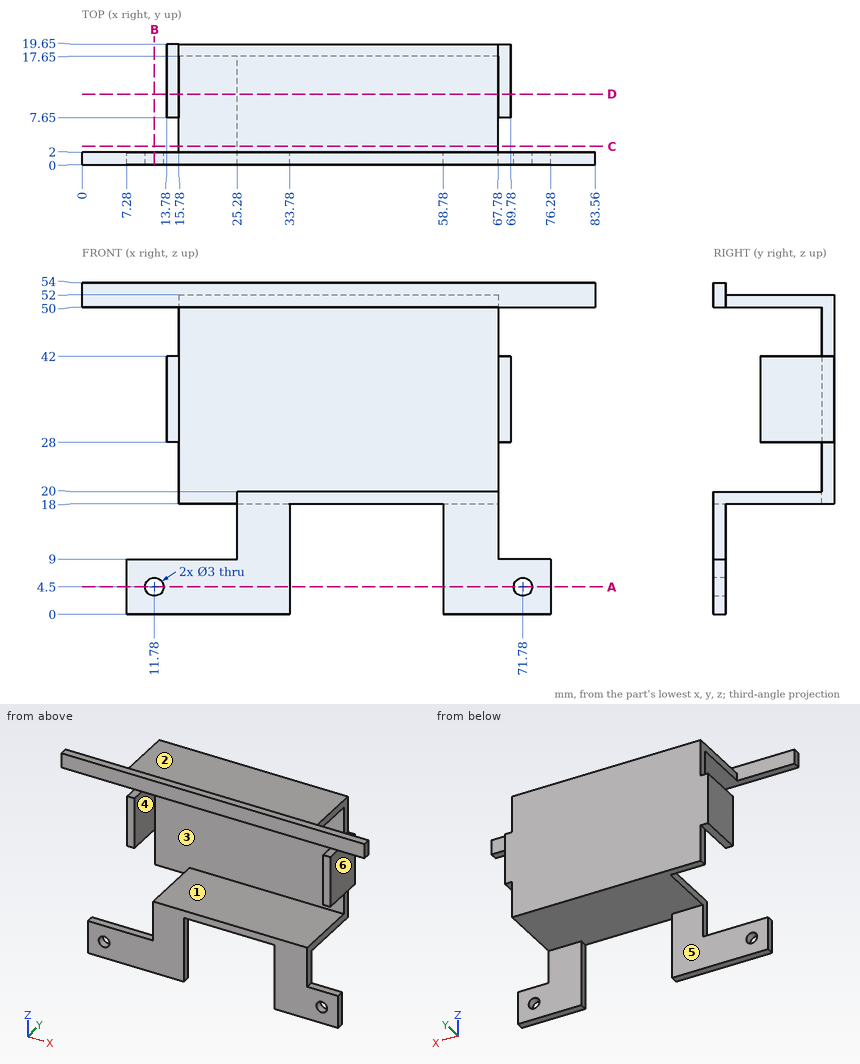
Design review of the part shown in the three views and the two pictorial views. Dimensions are in mm from the part's minimum x, y and z. A direction names the side the tool comes from. Coordinates: 2 decimals unless noted, no trailing zeros. Write each loop counter-clockwise with the first axis right and the second up, starting at its lowest first coordinate (ties: lowest second). Pieces come first, ordered by that corner, then holes.
(1) The part is to be moulded in two halves that separate along Z. For the marked faces 1, 2, 3 and 4, say which applies: +Z half, -Z half, draft (parallel to the pull), parting line (faces both ways), or undercut.
(2) Add section B-B on x = 11.78. Give the boundary of the cut face in (y, z), then the cut area to 3 significant figures.
(3) Add section D-D on y = 11.5. Give the boundary of the cut face in (x, z), then the cut area to 3 significant figures.
(4) Add section A-A on z = 4.5. Give the boundary of the cut face in (x, y).
(5) Add section C-C on y = 3. Give the boundary of the cut face in (x, z), then the cut area to 3 significant figures.
(6) Wall thickness on probe 1 along Z at (x, y) = (71.78, 1.1); probe 2 along X at (y, z) = (0.5, 4.5); probe 3 along Z at (x, y) = (14.5, 1): over which ranges is each line inside the solid? List them lowest first.
(7) Tool access review of the marked faces 5 and 6: name each direction out of +Z, -Z, +X, -X, +Y, -Y from which nothing blocks a thin tool from reaching the whole face with its end or side.
(8) For pin 1 Ø3 at (y, z) = (7, 35.5) entering from -X; pin 2 Ø6 at (x, z) = (18.5, 18) entering from -Y; pin 3 Ø2 at (x, z) = (14.5, 46.5) entering from +Y; pin 4 Ø2 at (x, z) = (15, 36) entering from -Y, all flat-tipped, find the tip position at first contact; note any pin that passes through.
Answer sheet:
1. face 1: undercut
1. face 2: +Z half
1. face 3: undercut
1. face 4: draft
2. outline: (0, 0) - (2, 0) - (2, 3) - (0, 3) - close; (0, 6) - (2, 6) - (2, 9) - (0, 9) - close; (0, 50) - (2, 50) - (2, 54) - (0, 54) - close
2. area: 20.0 mm2
3. outline: (13.78, 28) - (15.78, 28) - (15.78, 42) - (13.78, 42) - close; (15.78, 50) - (67.78, 50) - (67.78, 52) - (15.78, 52) - close; (25.28, 18) - (67.78, 18) - (67.78, 20) - (25.28, 20) - close; (67.78, 28) - (69.78, 28) - (69.78, 42) - (67.78, 42) - close
3. area: 245 mm2
4. outline: (7.28, 0) - (10.28, 0) - (10.28, 2) - (7.28, 2) - close; (13.28, 0) - (33.78, 0) - (33.78, 2) - (13.28, 2) - close; (58.78, 0) - (70.28, 0) - (70.28, 2) - (58.78, 2) - close; (73.28, 0) - (76.28, 0) - (76.28, 2) - (73.28, 2) - close
5. outline: (15.78, 50) - (67.78, 50) - (67.78, 52) - (15.78, 52) - close; (25.28, 18) - (67.78, 18) - (67.78, 20) - (25.28, 20) - close
5. area: 189 mm2
6. probe 1: z = 0 to 3, 6 to 9, 50 to 54
6. probe 2: x = 7.28 to 10.28, 13.28 to 33.78, 58.78 to 70.28, 73.28 to 76.28
6. probe 3: z = 0 to 9, 50 to 54
7. face 5: -Z, +X, -X, +Y
7. face 6: +Z, -Z, +X, +Y, -Y
8. pin 1: stops at x = 13.78
8. pin 2: stops at y = 17.65
8. pin 3: passes through
8. pin 4: stops at y = 7.65
